Work out the finished part from the listing and answer in its coordinate system (mm). A direction names the side the tool comes from. Give positions to 0.01 mm unless a question says otherwise; leave off trailing zeros. Order: outer loops, then holes, each group sorted by start corner. A loop starts at its lowest first (then second) coordinate and runs counter-clockwise, first axis right, second up. Notation, with made-up numbers: (81.5, 72.5) - (128.5, 72.5) arc R21 ccw to (128.5, 84.5) - close; hole circle Ø4 at (-30.75, -13). An arc over 180 degrees is marked (long way). Put each result on its own line as item: value.
```python
from build123d import *

# Parameters (mm, degrees)
SKETCH1_W           = 140
SKETCH1_H           = 92
SKETCH1_R           = 16.5
BOSS_EXTRUDE2_DEPTH = 15
SKETCH3_R           = 33
SKETCH3_R_2         = 21
BOSS_EXTRUDE3_DEPTH = 50
SKETCH4_RX          = 60
SKETCH4_RY          = 36
SKETCH4_R           = 6
SKETCH4_R_2         = 21
BOSS_EXTRUDE4_DEPTH = 15


with BuildPart() as part:
    # Sketch1 → Boss-Extrude2 (new body)
    with BuildSketch(Plane(origin=(0, 0, 0), x_dir=(1, 0, 0), z_dir=(0, 1, 0))):
        Rectangle(SKETCH1_W, SKETCH1_H)
        with Locations(Location((0, 0, 0), (0, 0, 270))):
            Circle(SKETCH1_R, mode=Mode.SUBTRACT)
    extrude(amount=BOSS_EXTRUDE2_DEPTH)

    # Sketch3 → Boss-Extrude3 (add)
    with BuildSketch(Plane(origin=(0, 15, 0), x_dir=(1, 0, 0), z_dir=(0, 1, 0))):
        with Locations(Location((0, 0, 0), (0, 0, 90))):
            Circle(SKETCH3_R)
        with Locations(Location((0, 0, 0), (0, 0, 270))):
            Circle(SKETCH3_R_2, mode=Mode.SUBTRACT)
    extrude(amount=BOSS_EXTRUDE3_DEPTH)

    # Sketch4 → Boss-Extrude4 (add)
    with BuildSketch(Plane(origin=(0, 65, 0), x_dir=(1, 0, 0), z_dir=(0, 1, 0))):
        with Locations((0, 0)):
            Ellipse(SKETCH4_RX, SKETCH4_RY)
        with Locations(Location((-42, 0, 0), (0, 0, 270))):
            Circle(SKETCH4_R, mode=Mode.SUBTRACT)
        with Locations(Location((42, 0, 0), (0, 0, 90))):
            Circle(SKETCH4_R, mode=Mode.SUBTRACT)
        with Locations(Location((0, 0, 0), (0, 0, 270))):
            Circle(SKETCH4_R_2, mode=Mode.SUBTRACT)
    extrude(amount=BOSS_EXTRUDE4_DEPTH)


solid = part.part
```
(1) Straight lines are drawn through the part: line 1 (X direction, y = 74, z = 0); line 2 (Y direction, x = 35.5, z = 13); line 3 (X direction, y = 69.5, z = -2). For each, find the intervals that lie inside material, in ascending order.
Geometry check:
line 1: x = -60 to -48, -36 to -21, 21 to 36, 48 to 60
line 2: y = 0 to 15, 65 to 80
line 3: x = -59.91 to -47.66, -36.34 to -20.9, 20.9 to 36.34, 47.66 to 59.91
(2) Section D-D, the plane y = 17.5 is taken. Write down the section's boundary in (x, z), then the cut area to 3 significant figures.
Geometry check:
outline: circle Ø66 at (0, 0); hole circle Ø42 at (0, 0)
area: 2,040 mm²
(3) Given pin 1 (1 mm diameter, centred on x = 10.5, y = 37, fed in from +Z); pin 2 (1 mm diameter, centred on y = 34.5, z = -28.5, fed in from +X); pin 3 (1 mm diameter, centred on x = -7, y = 63.5, fed in from -Z), each flat-ended and moving along its own axis, determine where each tip first touches the part or whether it passes through.
Geometry check:
pin 1: stops at z = 31.45
pin 2: stops at x = 17.46
pin 3: stops at z = -32.35
(4) A tool of negligible diameter and unlimited length cuts with its end or side. For faces 1 (the face through (-32, 15, -11)), 2 (the face through (70, 7, 1)), 3 (the face through (6.31, 47.04, 20.03)), from which of +Z, -Z, +X, -X, +Y, -Y can it reach the whole face along a straight path? Write none if from no direction.
Geometry check:
face 1: none
face 2: +Z, -Z, +X, +Y, -Y
face 3: +Y
(5) Section B-B, the plane x = -42 is taken. Count the separate pieces of the cut face and the enclosed holes in it, then the cut area to 3 significant figures.
Geometry check:
separate pieces: 3
enclosed holes: 0
area: 1,970 mm²
(6) Section A-A, the plane y = 8 is taken. Write down the section's boundary in (x, z).
Geometry check:
outline: (-70, -46) - (70, -46) - (70, 46) - (-70, 46) - close; hole circle Ø33 at (0, 0)
(7) Determine the mould class of faces 4 (the face through (-70, 7, 1)), 5 (the face through (-1, 7, -46)), 6 (the face through (-13, 15, 11)), 7 (the face through (47.857, 72.395, 1.301)) for opening direction Z: pulls with the +Z half, pulls with the -Z half, needs draft (parallel to the pull), parting line crosses it, or undercut.
Geometry check:
face 4: needs draft
face 5: pulls with the -Z half
face 6: undercut
face 7: undercut
